Check sheet for the modelled part. Datum: model origin and axes. Units: mm. Face numbers are marked on the shaded views. Coordinates: 2 decimals unless noted, no trailing zeros. Loops run counter-clockwise (first coordinate to the right, second up) from the corner with the lowest first, then second, coordinate; pieces in that order, holes last. Notation, with made-up numbers: (40, 55) -> (94, 55) arc R29 cw to (94, 82) -> close; hole circle Ø7 at (72.5, -29.75). An arc over 180 degrees is marked (long way). Use one line per item in the form item = value.
from build123d import *

# Parameters (mm, degrees)
SKETCH_1_W             = 120
SKETCH_1_H             = 80
EXTRUDE_1_DEPTH        = 15
SKETCH_2_R             = 25
CUT_EXTRUDE_1_DEPTH    = 15
SKETCH_3_R             = 5
CUT_EXTRUDE_2_DEPTH    = 15
PATTERN_LINEAR_1_COUNT = 3
PATTERN_LINEAR_1_PITCH = 30


with BuildPart() as part:
    # 草图1 → 凸台-拉伸1 (new body)
    with BuildSketch(Plane(origin=(0, 0, 0), x_dir=(1, 0, 0), z_dir=(0, 1, 0))):
        Rectangle(SKETCH_1_W, SKETCH_1_H)
    extrude(amount=EXTRUDE_1_DEPTH)

    # 草图2 → 切除-拉伸1 (cut)
    with BuildSketch(Plane(origin=(0, 0, 0), x_dir=(1, 0, 0), z_dir=(0, 1, 0))):
        with Locations(Location((0, 0, 0), (0, 0, 270))):
            Circle(SKETCH_2_R)
    extrude(amount=CUT_EXTRUDE_1_DEPTH, mode=Mode.SUBTRACT)

    # 草图3 → 切除-拉伸2 (cut)
    with BuildSketch(Plane(origin=(0, 0, 0), x_dir=(1, 0, 0), z_dir=(0, 1, 0))):
        with Locations(Location((40, 25, 0), (0, 0, 270))):
            Circle(SKETCH_3_R)
    cut_extrude_2 = extrude(amount=CUT_EXTRUDE_2_DEPTH, mode=Mode.SUBTRACT)

    # 阵列(线性)1: 切除-拉伸2 ×3
    with Locations(*[(-i * PATTERN_LINEAR_1_PITCH, 0, 0) for i in range(1, PATTERN_LINEAR_1_COUNT)]):
        add(cut_extrude_2, mode=Mode.SUBTRACT)


solid = part.part
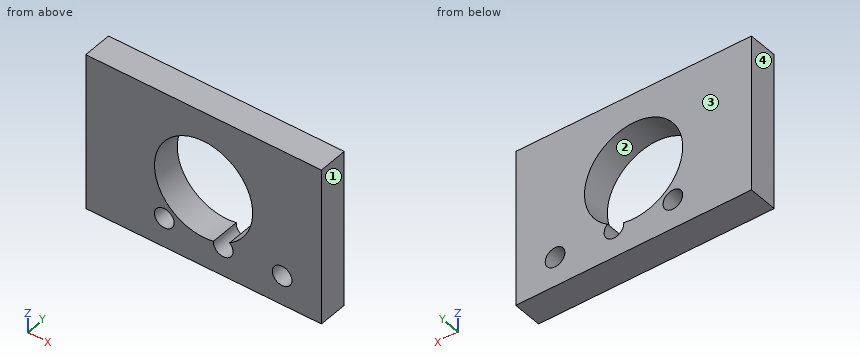
(1) Mould release check, pull along X, two halves, no side actions. Record for the marked faces 1, 2, 3 and 4: +X half, -X half, draft (parallel to the pull), parting line (faces both ways), or undercut.
Established:
face_1 = +X half
face_2 = undercut
face_3 = draft
face_4 = -X half
(2) Section check C-C, the plane z = -23. Record the boundary of the cut face in (x, y).
Established:
outline = (-60, 0) -> (-24.58, 0) -> (-24.58, 15) -> (-60, 15) -> close; (-15.42, 0) -> (-9.8, 0) -> (-9.8, 15) -> (-15.42, 15) -> close; (14.58, 0) -> (35.42, 0) -> (35.42, 15) -> (14.58, 15) -> close; (44.58, 0) -> (60, 0) -> (60, 15) -> (44.58, 15) -> close
(3) Section check D-D, the plane x = 0. Record the boundary of the cut face in (y, z), plus the area to 3 significant figures.
Established:
outline = (0, -40) -> (15, -40) -> (15, -25) -> (0, -25) -> close; (0, 25) -> (15, 25) -> (15, 40) -> (0, 40) -> close
area = 450 mm²
(4) Scan lines: line 1 along Z through (x, y) = (-17, 0.75); line 2 along Z through (x, y) = (0, 8.5); line 3 along X through (y, z) = (9.75, 1). Record each from-to range of solid material in increasing order.
Established:
line_1 = -40 to -29, -21 to -18.33, 18.33 to 40
line_2 = -40 to -25, 25 to 40
line_3 = -60 to -24.98, 24.98 to 60
(5) Section check B-B, the plane z = 0. Record the boundary of the cut face in (x, y).
Established:
outline = (-60, 0) -> (-25, 0) -> (-25, 15) -> (-60, 15) -> close; (25, 0) -> (60, 0) -> (60, 15) -> (25, 15) -> close
(6) Section check A-A, the plane x = -20. Record the boundary of the cut face in (y, z), plus the area to 3 significant figures.
Established:
outline = (0, -40) -> (15, -40) -> (15, -30) -> (0, -30) -> close; (0, -20) -> (15, -20) -> (15, -15) -> (0, -15) -> close; (0, 15) -> (15, 15) -> (15, 40) -> (0, 40) -> close
area = 600 mm²
